from build123d import *

# Parameters (mm, degrees)
BOSS_EXTRUDE1_DEPTH      = 3
BOSS_EXTRUDE1_DEPTH_BACK = 3
SKETCH1_R                = 1
CUT_EXTRUDE1_DEPTH       = 1.6
CUT_EXTRUDE1_DEPTH_BACK  = 1.6
SKETCH2_R                = 7.5
CUT_EXTRUDE2_DEPTH       = 0.7
CUT_EXTRUDE2_DEPTH_BACK  = 0.7
SKETCH3_R                = 7.5


with BuildPart() as part:
    # Sketch1 → Boss-Extrude1 (new, two sides: drawn at the far end of the back side and taken through both)
    with BuildSketch(Plane.XY.offset(-BOSS_EXTRUDE1_DEPTH_BACK)):
        with BuildLine():
            ThreePointArc((-2.25, 0), (0, -2.25), (2.25, 0))
            ThreePointArc((2.25, 0), (21, 18.75), (39.75, 0))
            ThreePointArc((39.75, 0), (42, -2.25), (44.25, 0))
            ThreePointArc((44.25, 0), (21, 23.25), (-2.25, 0))
        make_face()
        Circle(SKETCH1_R, mode=Mode.SUBTRACT)
        with Locations((42, 0)):
            Circle(SKETCH1_R, mode=Mode.SUBTRACT)
    extrude(amount=BOSS_EXTRUDE1_DEPTH + BOSS_EXTRUDE1_DEPTH_BACK)

    # Sketch2 → Cut-Extrude1 (cut, two sides: drawn at the far end of the back side and taken through both)
    with BuildSketch(Plane.XY.offset(-CUT_EXTRUDE1_DEPTH_BACK)):
        Circle(SKETCH2_R)
    extrude(amount=CUT_EXTRUDE1_DEPTH + CUT_EXTRUDE1_DEPTH_BACK, mode=Mode.SUBTRACT)

    # Sketch3 → Cut-Extrude2 (cut, two sides: drawn at the far end of the back side and taken through both)
    with BuildSketch(Plane.XY.offset(-CUT_EXTRUDE2_DEPTH_BACK)):
        with Locations((42, 0)):
            Circle(SKETCH3_R)
    extrude(amount=CUT_EXTRUDE2_DEPTH + CUT_EXTRUDE2_DEPTH_BACK, mode=Mode.SUBTRACT)


solid = part.part
Verification items for the finished model (mm, model axes). A direction names the side the tool comes from. Give positions to 0.01 mm unless a question says otherwise; leave off trailing zeros. Loops run counter-clockwise (first coordinate to the right, second up) from the corner with the lowest first, then second, coordinate; pieces in that order, holes last.
1) Set-up check for faces 1 (the cylindrical face through (1.311, 7.384, -0.022)), 2 (the cylindrical face through (20.588, 18.745, -0.042)): record each of +Z, -Z, +X, -X, +Y, -Y from which the full face is reachable in a straight line by a thin tool's end or side.
2) Depth check by flat-ended pin: pin 1 Ø3 at (x, z) = (12.5, 2) entering from -Y; pin 2 Ø3 at (x, y) = (6, 3.5) entering from +Z; pin 3 Ø3 at (y, z) = (10.5, -0.5) entering from -X; pin 4 Ø1 at (x, z) = (8, -1) entering from +Y. Enter the tip coordinate at first touch or a pass-through.
3) Sectioned sample at D-D, the plane y = 14.75. Enter the section's corners in (x, z).
4) Sectioned sample at A-A, the plane y = 11.75. Enter the section's corners in (x, z), then the cut area to 3 significant figures.
5) Thickness scan on line 1 along X through (y, z) = (7.5, -2.15); line 2 along Y through (x, z) = (42, -1.4); line 3 along Y through (x, z) = (21, -2.05). Record the ranges inside material, lowest first.
6) Sectioned sample at B-B, the plane z = -2.45. Enter the section's corners in (x, y).
7) Sectioned sample at C-C, the plane x = 42. Enter the section's corners in (y, z), then the cut area to 3 significant figures.
8) Draft check along Z on faces 3 (the cylindrical face through (-0.05, -2.25, -2.31)), 4 (the flat face through (1, 3, 1.6)), 5 (the flat face through (21, 19, 3)), 6 (the flat face through (21, 19, -3)). Enter one of: pulls with the +Z half, pulls with the -Z half, needs draft (parallel to the pull), parting line crosses it, or undercut.
Answers:
1. face 1: -Y
1. face 2: +Z, -Z, -Y
2. pin 1: stops at y = 15.86
2. pin 2: passes through
2. pin 3: stops at x = -0.44
2. pin 4: stops at y = 19.6
3. outline: (3.03, -3) - (9.42, -3) - (9.42, 3) - (3.03, 3) - close; (32.58, -3) - (38.97, -3) - (38.97, 3) - (32.58, 3) - close
4. outline: (0.94, -3) - (6.39, -3) - (6.39, 3) - (0.94, 3) - close; (35.61, -3) - (41.06, -3) - (41.06, 3) - (35.61, 3) - close
4. area: 65.4 mm2
5. line 1: x = -1.01 to 3.82, 38.18 to 43.01
5. line 2: y = -2.25 to -1, 1 to 9.98
5. line 3: y = 18.75 to 23.25
6. outline: (-2.25, 0) arc R2.25 ccw to (2.25, 0) arc R18.75 cw to (39.75, 0) arc R2.25 ccw to (44.25, 0) arc R23.25 ccw to start; hole circle Ø2 at (0, 0); hole circle Ø2 at (42, 0)
7. outline: (-2.25, -3) - (-1, -3) - (-1, -0.7) - (-2.25, -0.7) - close; (-2.25, 0.7) - (-1, 0.7) - (-1, 3) - (-2.25, 3) - close; (1, -3) - (9.98, -3) - (9.98, 3) - (1, 3) - (1, 0.7) - (7.5, 0.7) - (7.5, -0.7) - (1, -0.7) - close
7. area: 50.5 mm2
8. face 3: needs draft
8. face 4: undercut
8. face 5: pulls with the +Z half
8. face 6: pulls with the -Z half
